Geometry: final body of the model. Coordinates: model frame, mm. A direction names the side the tool comes from. Give positions to 0.01 mm unless a question says otherwise; leave off trailing zeros. Order: outer loops, then holes, each group sorted by start corner. A loop starts at its lowest first (then second) coordinate and runs counter-clockwise, first axis right, second up. Notation, with made-up numbers: (37, 83) -> (46, 83) arc R14 ccw to (46, 96) -> close; hole circle Ø1 at (88, 61). An arc over 180 degrees is marked (long way). Answer in a Markdown table with one row per item. Add a question column.
Q1. Cut plane B-B on y = -12.5. Return the cut outline in (x, z), and give its area (3 significant figures).
Q2. Cut plane C-C on y = -39.5. Return the cut outline in (x, z).
Q3. Pull-direction query (X, two-part tool) for faces 1 (the face through (0.28, 53.29, 1.45)), 2 (the face through (-37.409, -1, 13)), 3 (the face through (0, -63.977, 13)); classes: +X half, -X half, draft (parallel to the pull), parting line (faces both ways), or undercut.
Q4. Cut plane A-A on x = -2.5. Return the cut outline in (y, z), and give its area (3 significant figures).
Q5. Set-up query: faces 4 (the face through (0.28, -53.29, 1.45)), 5 (the face through (-0.28, 53.29, 23.95)), 6 (the face through (31, 13, 0)), 7 (the face through (-24.889, -1, 13)). Return all of +Z, -Z, +X, -X, +Y, -Y with unobstructed straight access to the full face (end or side cutting, diameter ignored); none if empty.
Q6. Line query: line 1 along Y through (x, z) = (-15, 18); line 2 along X through (y, z) = (6, 13.25); line 3 along Y through (x, z) = (25, 23). Output: solid intervals per line, ascending. Write a range as from..to.
Q7. Contact query for flat-ended pins moving along their axis: P1, Ø6, axis at x = -22.5, y = -8.5, coming from the -Z side; P2, Ø8, axis at y = -42.6, z = 12.37, coming from the +X side; P3, Ø1.5, axis at x = 20.5, z = 4, coming from the -Y side; P4, Ø10, axis at x = 23.5, y = 35, coming from the +Z side. Output: stop coordinate, or through.
from build123d import *

# Parameters (mm, degrees)
F0_W     = 74.8185142875
F0_H     = 127.9549151659
F1_DEPTH = 25.4
F2_W     = 49.7772097588
F2_H     = 103.5243868828
F3_DEPTH = 38.1
F4_R     = 5.08
F5_R     = 4.9743780925
F6_DEPTH = 127
F7_R     = 5.0201571666
F8_DEPTH = 127


with BuildPart() as f1:
    # F0 (on Top) → F1 (new body)
    with BuildSketch(Plane.XY):
        Rectangle(F0_W, F0_H)
    extrude(amount=F1_DEPTH)

    # F2 (on Top) → F3 (cut)
    with BuildSketch(Plane.XY):
        Rectangle(F2_W, F2_H)
    extrude(amount=F3_DEPTH, mode=Mode.SUBTRACT)

    # F4
    f4_edges = [f1.edges().sort_by_distance(p)[0] for p in [
        (37.409257, 63.977458, 12.7),
        (-37.409257, 63.977458, 12.7),
        (0, 63.977458, 0),
        (0, 63.977458, 25.4),
        (37.409257, 0, 25.4),
        (0, -63.977458, 25.4),
        (-37.409257, 0, 25.4),
        (0, 51.762193, 25.4),
        (-24.888605, 0, 25.4),
        (0, -51.762193, 25.4),
        (24.888605, 0, 25.4),
        (-37.409257, -63.977458, 12.7),
        (-37.409257, 0, 0),
        (37.409257, -63.977458, 12.7),
        (0, -63.977458, 0),
        (37.409257, 0, 0),
        (-24.888605, 0, 0),
        (-24.888605, -51.762193, 12.7),
        (-24.888605, 51.762193, 12.7),
        (24.888605, 0, 0),
        (24.888605, 51.762193, 12.7),
        (24.888605, -51.762193, 12.7),
        (0, -51.762193, 0),
        (0, 51.762193, 0),
    ]]
    fillet(f4_edges, radius=F4_R)

    # F5 (on face) → F6 (cut)
    with BuildSketch(Plane.YZ.offset(37.4092571437)):
        with Locations((-42.6007434726, 12.3679572716)):
            Circle(F5_R)
    extrude(amount=-F6_DEPTH, mode=Mode.SUBTRACT)

    # F7 (on face) → F8 (cut)
    with BuildSketch(Plane.YZ.offset(37.4092571437)):
        with Locations((40.1576943696, 12.6733398065)):
            Circle(F7_R)
    extrude(amount=-F8_DEPTH, mode=Mode.SUBTRACT)


solid = f1.part
Completed:
| question | item | result |
|---|---|---|
| 1 | outline | (-37.41, 5.08) arc R5.08 ccw to (-32.33, 0) -> (-29.97, 0) arc R5.08 ccw to (-24.89, 5.08) -> (-24.89, 20.32) arc R5.08 ccw to (-29.97, 25.4) -> (-32.33, 25.4) arc R5.08 ccw to (-37.41, 20.32) -> close; (24.89, 5.08) arc R5.08 ccw to (29.97, 0) -> (32.33, 0) arc R5.08 ccw to (37.41, 5.08) -> (37.41, 20.32) arc R5.08 ccw to (32.33, 25.4) -> (29.97, 25.4) arc R5.08 ccw to (24.89, 20.32) -> close |
| 1 | area | 592 mm² |
| 2 | outline | (-37.41, 5.08) arc R5.08 ccw to (-32.33, 0) -> (-29.97, 0) arc R5.08 ccw to (-24.89, 5.08) -> (-24.89, 8.48) -> (-37.41, 8.48) -> close; (-37.41, 16.26) -> (-24.89, 16.26) -> (-24.89, 20.32) arc R5.08 ccw to (-29.97, 25.4) -> (-32.33, 25.4) arc R5.08 ccw to (-37.41, 20.32) -> close; (24.89, 5.08) arc R5.08 ccw to (29.97, 0) -> (32.33, 0) arc R5.08 ccw to (37.41, 5.08) -> (37.41, 8.48) -> (24.89, 8.48) -> close; (24.89, 16.26) -> (37.41, 16.26) -> (37.41, 20.32) arc R5.08 ccw to (32.33, 25.4) -> (29.97, 25.4) arc R5.08 ccw to (24.89, 20.32) -> close |
| 3 | face 1 | undercut |
| 3 | face 2 | -X half |
| 3 | face 3 | draft |
| 4 | outline | (-63.98, 5.08) arc R5.08 ccw to (-58.9, 0) -> (-56.84, 0) arc R5.08 ccw to (-51.76, 5.08) -> (-51.76, 20.32) arc R5.08 ccw to (-56.84, 25.4) -> (-58.9, 25.4) arc R5.08 ccw to (-63.98, 20.32) -> close; (51.76, 5.08) arc R5.08 ccw to (56.84, 0) -> (58.9, 0) arc R5.08 ccw to (63.98, 5.08) -> (63.98, 20.32) arc R5.08 ccw to (58.9, 25.4) -> (56.84, 25.4) arc R5.08 ccw to (51.76, 20.32) -> close |
| 4 | area | 576 mm² |
| 5 | face 4 | -Z |
| 5 | face 5 | +Z |
| 5 | face 6 | -Z, +X, -X, +Y, -Y |
| 5 | face 7 | +Z, -Z |
| 6 | line 1 | y = -63.98..-51.76, 51.76..63.98 |
| 6 | line 2 | x = -37.41..-24.89, 24.89..37.41 |
| 6 | line 3 | y = -63.21..-49.37, 49.37..63.21 |
| 7 | P1 | stops at z = 2.66 |
| 7 | P2 | passes through |
| 7 | P3 | stops at y = -63.97 |
| 7 | P4 | stops at z = 25.18 |
